from build123d import *

# Parameters (mm, degrees)
SALIENTE_EXTRUIR1_DEPTH = 10
CROQUIS2_R              = 10
CORTAR_EXTRUIR1_DEPTH   = 10
CROQUIS3_W              = 25
CROQUIS3_H              = 58
CORTAR_EXTRUIR2_DEPTH   = 5


with BuildPart() as part:
    # Croquis1 → Saliente-Extruir1 (new body)
    with BuildSketch(Plane(origin=(0, 0, 0), x_dir=(1, 0, 0), z_dir=(0, 1, 0))):
        Polygon((-86.291306126, 50.535240052), (-86.910454734, -49.462843205), (-0.619148608, -99.998083257), (86.291306126, -50.535240052), (86.910454734, 49.462843205), (0.619148608, 99.998083257), align=None)
    extrude(amount=SALIENTE_EXTRUIR1_DEPTH)

    # Croquis2 → Cortar-Extruir1 (cut)
    with BuildSketch(Plane(origin=(0, 10, 0), x_dir=(1, 0, 0), z_dir=(0, 1, 0))):
        with Locations(Location((0, 0, 0), (0, 0, 270))):
            Circle(CROQUIS2_R)
    extrude(amount=-CORTAR_EXTRUIR1_DEPTH, mode=Mode.SUBTRACT)

    # Croquis3 → Cortar-Extruir2 (cut)
    with BuildSketch(Plane(origin=(0, 10, 0), x_dir=(1, 0, 0), z_dir=(0, 1, 0))):
        with Locations((48.693290604, -13.979093197)):
            Rectangle(CROQUIS3_W, CROQUIS3_H)
    extrude(amount=-CORTAR_EXTRUIR2_DEPTH, mode=Mode.SUBTRACT)


solid = part.part
CAD build for the part. Positions are in the model's coordinates, mm. A direction names the side the tool comes from. Round coordinates to 2 decimals unless told otherwise and drop trailing zeros. Loops run counter-clockwise (first coordinate to the right, second up) from the corner with the lowest first, then second, coordinate; pieces in that order, holes last. Notation, with made-up numbers: (-8.5, 19.5) - (40.5, 19.5) arc R38 cw to (40.5, 58.5) - close; hole circle Ø8 at (77.25, 10). An arc over 180 degrees is marked (long way). Put each result on its own line as item: value.
1. Slice it at A-A on x = 4. List the corners of the cut face in (y, z), and give its area (3 significant figures).
Geometry check:
outline: (0, -98.02) - (10, -98.02) - (10, -9.17) - (0, -9.17) - close; (0, 9.17) - (10, 9.17) - (10, 97.37) - (0, 97.37) - close
area: 1,770 mm²
2. Wall check: line 1 (X direction, y = 5.75, z = 0); line 2 (X direction, y = 1, z = 49); line 3 (Z direction, x = 41, y = 9.25). Give the ranges that are in metal, low to high.
Geometry check:
line 1: -86.6 to -10, 10 to 36.19, 61.19 to 86.6
line 2: -86.91 to 86.3
line 3: -76.35 to -15.02, 42.98 to 76.31
3. Two-plate mould, pull along Z, no slides. Class faces 1 (the flat face through (49, 5, 14)), 2 (the flat face through (49, 8, -15.021)), 3 (the flat face through (44.369, 4.93, -74.377)), 4 (the flat face through (-44.369, 4.93, 74.377)): released by +Z, released by -Z, zero draft, split by the parting line, or undercut.
Geometry check:
face 1: undercut
face 2: undercut
face 3: released by -Z
face 4: released by +Z
4. Slice it at B-B on y = 2.5. List the corners of the cut face in (x, z).
Geometry check:
outline: (-86.91, 49.46) - (-86.29, -50.54) - (0.62, -100) - (86.91, -49.46) - (86.29, 50.54) - (-0.62, 100) - close; hole circle Ø20 at (0, 0)
5. Slice it at D-D on x = 29. List the corners of the cut face in (y, z).
Geometry check:
outline: (0, -83.38) - (10, -83.38) - (10, 83.14) - (0, 83.14) - close
6. 3-axis set-ups, long thin cutter, end or side, ignore diameter. For faces 5 (the flat face through (-21, 10, -1)), 6 (the flat face through (36.193, 8, 14)): which of +Z, -Z, +X, -X, +Y, -Y reach the whole face in a straight line?
Geometry check:
face 5: +Z, -Z, +X, -X, +Y
face 6: +Y
7. Slice it at C-C on z = 0. List the corners of the cut face in (x, y).
Geometry check:
outline: (-86.6, 0) - (-10, 0) - (-10, 10) - (-86.6, 10) - close; (10, 0) - (86.6, 0) - (86.6, 10) - (61.19, 10) - (61.19, 5) - (36.19, 5) - (36.19, 10) - (10, 10) - close
8. Pin check, flat tips, straight feed: P1, Ø2, axis at x = -57.5, y = 7, coming from the -Z side; P2, Ø7.5, axis at x = 50, z = 0, coming from the +Y side; P3, Ø6, axis at x = -39.5, y = 7.5, coming from the -Z side. Stop position of each tip, or through.
Geometry check:
P1: z = -67.49
P2: y = 5
P3: z = -78.87
